Here's how the part is built. I have some questions about the finished solid (model axes, mm). A direction names the side the tool comes from. Coordinates: 2 decimals unless noted, no trailing zeros. Write each loop counter-clockwise with the first axis right and the second up, starting at its lowest first coordinate (ties: lowest second). Pieces come first, ordered by that corner, then holes. Notation, with made-up numbers: (27, 37) -> (31, 37) arc R28 cw to (31, 65) -> close; hole circle Ø10 at (-22.75, -40). An arc over 180 degrees is marked (long way). Use a Markdown table: item, result. Add a question column.
```python
from build123d import *

# Parameters (mm, degrees)
BOSS_EXTRUDE1_DEPTH             = 60
BOSS_EXTRUDE2_REACH             = 90.732
SKETCH5_W                       = 5
SKETCH5_H                       = 7.5
BOSS_EXTRUDE2_DIRECTION_2_DEPTH = 15
FILLET1_R                       = 1.5
CUT_EXTRUDE1_REACH              = 75.969
SKETCH6_R                       = 1


# Read off the part's stored shape, not the designer's step: Boss-Extrude1
with BuildPart() as part:
    # Boss-Extrude1 outline → Boss-Extrude1 (new body)
    with BuildSketch(Plane(origin=(0, 0, 0), x_dir=(0, 0, -1), z_dir=(1, 0, 0))):
        Polygon((45.19977735, 6.923160404), (48.514979298, 2.188561349), (50.553744228, 2.192162497), (51.753724693, 2.204282084), (56.563717189, 2.212778158), (57.763697654, 2.224897745), (61.363692038, 2.231256553), (62.563672503, 2.24337614), (64.963668759, 2.247615346), (65.19977735, 2.25), (64.373245759, 2.486572833), (63.782964065, 2.645530446), (63.182682388, 2.804470395), (62.592400694, 2.963428007), (61.401837323, 3.281325569), (60.211291616, 3.589223146), (56.639707483, 4.482915924), (55.439214781, 4.760795885), (53.058229346, 5.316591132), (50.677314564, 5.832386443), (48.296435109, 6.328181784), (47.09601306, 6.566061807), (45.905608659, 6.793959509), align=None)
    extrude(amount=BOSS_EXTRUDE1_DEPTH)

    # Sketch5 → Boss-Extrude2 (add, up to next)
    with BuildSketch(Plane(origin=(0, 2.188561349, 0), x_dir=(1, 0, 0), z_dir=(0, 1, 0)), mode=Mode.PRIVATE) as boss_extrude2_sk1:
        with Locations((30, 52.264979298)):
            Rectangle(SKETCH5_W, SKETCH5_H)
    boss_extrude2_tool1 = extrude(boss_extrude2_sk1.sketch, amount=BOSS_EXTRUDE2_REACH, mode=Mode.PRIVATE) - part.part
    add(boss_extrude2_tool1.solids().sort_by_distance((30, 2.188561, -52.264979))[0])

    # Sketch5 → Boss-Extrude2 direction 2 (add)
    with BuildSketch(Plane(origin=(0, 2.188561349, 0), x_dir=(1, 0, 0), z_dir=(0, 1, 0))):
        with Locations((30, 52.264979298)):
            Rectangle(SKETCH5_W, SKETCH5_H)
    extrude(amount=-BOSS_EXTRUDE2_DIRECTION_2_DEPTH)

    # Fillet1
    fillet1_edges = [part.edges().sort_by_distance(p)[0] for p in [
        (27.5, -5.311438651, -48.514979298),
        (27.5, -12.811438651, -52.264979298),
        (27.5, -5.299814875, -56.014979298),
        (30, -12.811438651, -56.014979298),
        (32.5, -5.299814875, -56.014979298),
        (32.5, -12.811438651, -52.264979298),
        (30, -12.811438651, -48.514979298),
        (32.5, -5.311438651, -48.514979298),
    ]]
    fillet(fillet1_edges, radius=FILLET1_R)

    # Sketch6 → Cut-Extrude1 (cut, up to next)
    with BuildSketch(Plane.ZY.offset(-27.5), mode=Mode.PRIVATE) as cut_extrude1_sk1:
        with Locations((-52.264979298, -7.311438651)):
            Circle(SKETCH6_R)
    cut_extrude1_tool1 = extrude(cut_extrude1_sk1.sketch, amount=-CUT_EXTRUDE1_REACH, mode=Mode.PRIVATE) & part.part
    # Sketch6 → Cut-Extrude1 (cut, up to next)
    with BuildSketch(Plane.ZY.offset(-27.5), mode=Mode.PRIVATE) as cut_extrude1_sk2:
        with Locations((-52.264979298, -2.311438651)):
            Circle(SKETCH6_R)
    cut_extrude1_tool2 = extrude(cut_extrude1_sk2.sketch, amount=-CUT_EXTRUDE1_REACH, mode=Mode.PRIVATE) & part.part
    add(cut_extrude1_tool1.solids().sort_by_distance((27.5, -7.311439, -52.264979))[0], mode=Mode.SUBTRACT)
    add(cut_extrude1_tool2.solids().sort_by_distance((27.5, -2.311439, -52.264979))[0], mode=Mode.SUBTRACT)


solid = part.part
```
Q1. Thinking about a two-plate mould opening in Y: for faces 1 (the cylindrical face through (29.96, -7.01, -51.31)), 2 (the flat face through (60, 4, -53)), 3 (the flat face through (29.58, 3.12, -62.01)), 4 (the flat face through (30, -12.811, -52)), which applies, released by +Y, released by -Y, zero draft, split by the parting line, or undercut?
Q2. Suppose I cut it at A-A, the plane y = -5.5. Write out the boundary of the cut face in (x, z), and give its area (3 significant figures).
Q3. Which directions (+Z, -Z, +X, -X, +Y, -Y) give clear straight access to the entire face, cutting with the end or side of a thin tool? Please do faces 5 (the flat face through (27.5, -4, -52)), 6 (the flat face through (32.5, -4, -52)), 7 (the flat face through (29.58, 6.077, -49.504)), 8 (the cylindrical face through (27.928, -4.655, -48.966)).
Q4. Suppose I cut it at B-B, the plane x = 37.5. Write out the boundary of the cut face in (y, z).
Q5. Will these pins go through, and if not, where does the flat tip stop? pin 1 (2 mm diameter, centred on x = 30.5, y = -2, fed in from -Z) (3 decimals); pin 2 (5 mm diameter, centred on y = -3, z = -51.5, fed in from +X); pin 3 (12 mm diameter, centred on x = 48, z = -51, fed in from -Y); pin 4 (6 mm diameter, centred on x = 22.5, y = -4.5, fed in from -Z).
Q6. Please list where these lines run through material, in increasing order: line 1 (X direction, y = -2.5, z = -50.75); line 2 (Y direction, x = 14.5, z = -60.5); line 3 (Y direction, x = 55.5, z = -62.25).
Q7. Suppose I cut it at C-C, the plane z = -59. Write out the boundary of the cut face in (x, y), and give its area (3 significant figures).
Answer key:
| question | item | result |
|---|---|---|
| 1 | face 1 | undercut |
| 1 | face 2 | zero draft |
| 1 | face 3 | released by +Y |
| 1 | face 4 | released by -Y |
| 2 | outline | (27.5, -54.51) arc R1.5 ccw to (29, -56.01) -> (31, -56.01) arc R1.5 ccw to (32.5, -54.51) -> (32.5, -50.01) arc R1.5 ccw to (31, -48.51) -> (29, -48.51) arc R1.5 ccw to (27.5, -50.01) -> close |
| 2 | area | 35.6 mm^2 |
| 3 | face 5 | +Z, -Z, -X, -Y |
| 3 | face 6 | +Z, -Z, +X, -Y |
| 3 | face 7 | -Z, +X, -X, +Y |
| 3 | face 8 | +Z, -X, -Y |
| 4 | outline | (2.19, -50.55) -> (2.2, -51.75) -> (2.21, -56.56) -> (2.22, -57.76) -> (2.23, -61.36) -> (2.24, -62.56) -> (2.25, -64.96) -> (2.25, -65.2) -> (2.49, -64.37) -> (2.65, -63.78) -> (2.8, -63.18) -> (2.96, -62.59) -> (3.28, -61.4) -> (3.59, -60.21) -> (4.48, -56.64) -> (4.76, -55.44) -> (5.32, -53.06) -> (5.83, -50.68) -> (6.33, -48.3) -> (6.57, -47.1) -> (6.79, -45.91) -> (6.92, -45.2) -> (2.19, -48.51) -> close |
| 5 | pin 1 | stops at z = -56.015 |
| 5 | pin 2 | stops at x = 32.5 |
| 5 | pin 3 | stops at y = 2.19 |
| 5 | pin 4 | passes through |
| 6 | line 1 | x = 27.5 to 32.5 |
| 6 | line 2 | y = 2.23 to 3.51 |
| 6 | line 3 | y = 2.24 to 3.05 |
| 7 | outline | (0, 2.23) -> (60, 2.23) -> (60, 3.89) -> (0, 3.89) -> close |
| 7 | area | 99.9 mm^2 |
